Could you check a few things on this model? Use its own coordinates, in mm. A direction names the side the tool comes from. Give positions to 0.01 mm unless a question says otherwise; leave off trailing zeros. Write each loop counter-clockwise with the first axis right and the second up, starting at its lowest first coordinate (ties: lowest second). Pieces come first, ordered by that corner, then holes. Notation, with made-up numbers: (59, 73) - (111, 73) arc R31 ccw to (111, 99) - close; hole circle Ø5 at (-1.5, 28.25). An arc over 180 degrees is marked (long way). Answer as a JSON object with one key per item and string values. Group by question number.
```python
from build123d import *

# Parameters (mm, degrees)
SKETCH_1_W          = 140
SKETCH_1_H          = 55
EXTRUDE_1_DEPTH     = 12
SKETCH_2_R          = 6.5
SKETCH_2_R_2        = 4.5
CUT_EXTRUDE_1_DEPTH = 77.159372371
FILLET_1_R          = 3
SKETCH_10_R         = 7
CUT_EXTRUDE_2_DEPTH = 8
SKETCH_11_R         = 15
CUT_EXTRUDE_3_DEPTH = 8
HOLE_WIZARD_M6_1_D  = 5


with BuildPart() as part:
    # 草图1 → 凸台-拉伸1 (new body)
    with BuildSketch(Plane.XY):
        Rectangle(SKETCH_1_W, SKETCH_1_H)
    extrude(amount=EXTRUDE_1_DEPTH)

    # 草图2 → 切除-拉伸1 (cut, through all)
    with BuildSketch(Plane.XY.offset(12)):
        Circle(SKETCH_2_R)
        with Locations((-53, 0)):
            Circle(SKETCH_2_R_2)
        with Locations((53, 0)):
            Circle(SKETCH_2_R_2)
    extrude(amount=-CUT_EXTRUDE_1_DEPTH, mode=Mode.SUBTRACT)

    # 圆角1
    fillet_1_edges = [part.edges().sort_by_distance(p)[0] for p in [
        (70, -27.5, 6),
        (-70, -27.5, 6),
        (-70, 27.5, 6),
        (70, 27.5, 6),
    ]]
    fillet(fillet_1_edges, radius=FILLET_1_R)

    # 草图10 → 切除-拉伸2 (cut)
    with BuildSketch(Plane.XY.offset(12)):
        with Locations((-53, 0)):
            Circle(SKETCH_10_R)
        with Locations((53, 0)):
            Circle(SKETCH_10_R)
    extrude(amount=-CUT_EXTRUDE_2_DEPTH, mode=Mode.SUBTRACT)

    # 草图11 → 切除-拉伸3 (cut)
    with BuildSketch(Plane.XY.offset(12)):
        Circle(SKETCH_11_R)
    extrude(amount=-CUT_EXTRUDE_3_DEPTH, mode=Mode.SUBTRACT)

    # M6 螺纹孔1 (through all)
    with Locations(Plane.XY.offset(12)):
        with Locations((-60, 22.5), (-60, -22.5), (0, -22.5), (0, 22.5), (60, 22.5), (60, -22.5)):
            Hole(HOLE_WIZARD_M6_1_D / 2)


solid = part.part
```
(1) I want a section at C-C, the plane x = -53. Please give me the cut outline in (y, z).
(2) I want a section at A-A, the plane y = 22.5. Please give me the cut outline in (x, z).
(3) I want a section at D-D, the plane y = 0. Please give me the cut outline in (x, z), and give its area (3 significant figures).
(4) I want a section at B-B, the plane z = 8.5. State how many separate pieces and enclosed holes the cut face has, and give its area (3 significant figures).
(5) I need wall thicknesses on L1, parallel to Y at x = 0, z = 1.6; L2, parallel to Y at x = 0, z = 5.75; L3, parallel to Y at x = 60, z = 2.5. Which ranges of each line are inside material? Lowest first, please.
(6) Will these pins go through, and if not, where does the flat tip stop? P1, Ø8, axis at x = 50, y = 7.5, coming from the -Z side; P2, Ø4.5, axis at x = -60, y = -22.5, coming from the -Z side; P3, Ø24, axis at x = 1.5, y = 2.5, coming from the +Z side.
(7) If we mould it in two halves opening along Y, with no side actions, what happens to faces 1 (the flat face through (-1, 27.5, 6)), 2 (the cylindrical face through (58.66, -20.39, 5.92)), 3 (the cylindrical face through (69.1, -26.64, 6.08))? For each: +Y half, -Y half, draft (parallel to the pull), parting line (faces both ways), or undercut.
(8) For faces 4 (the flat face through (-53, -5, 4)), 5 (the cylindrical face through (-61.34, -20.39, 5.92)), which set-ups out of +Z, -Z, +X, -X, +Y, -Y let a thin tool reach every point of the face, with its end or its side?
Entries:
{
 "1": {"outline": "(-27.5, 0) - (-4.5, 0) - (-4.5, 4) - (-7, 4) - (-7, 12) - (-27.5, 12) - close; (4.5, 0) - (27.5, 0) - (27.5, 12) - (7, 12) - (7, 4) - (4.5, 4) - close"},
 "2": {"outline": "(-70, 0) - (-62.5, 0) - (-62.5, 12) - (-70, 12) - close; (-57.5, 0) - (-2.5, 0) - (-2.5, 12) - (-57.5, 12) - close; (2.5, 0) - (57.5, 0) - (57.5, 12) - (2.5, 12) - close; (62.5, 0) - (70, 0) - (70, 12) - (62.5, 12) - close"},
 "3": {"outline": "(-70, 0) - (-57.5, 0) - (-57.5, 4) - (-60, 4) - (-60, 12) - (-70, 12) - close; (-48.5, 0) - (-6.5, 0) - (-6.5, 4) - (-15, 4) - (-15, 12) - (-46, 12) - (-46, 4) - (-48.5, 4) - close; (6.5, 0) - (48.5, 0) - (48.5, 4) - (46, 4) - (46, 12) - (15, 12) - (15, 4) - (6.5, 4) - close; (57.5, 0) - (70, 0) - (70, 12) - (60, 12) - (60, 4) - (57.5, 4) - close", "area": "1,090 mm^2"},
 "4": {"separate pieces": "1", "enclosed holes": "9", "area": "6,560 mm^2"},
 "5": {"L1": "-27.5 to -25, -20 to -6.5, 6.5 to 20, 25 to 27.5", "L2": "-27.5 to -25, -20 to -15, 15 to 20, 25 to 27.5", "L3": "-27.5 to -25, -20 to 20, 25 to 27.5"},
 "6": {"P1": "z = 0", "P2": "through", "P3": "z = 4"},
 "7": {"face 1": "+Y half", "face 2": "undercut", "face 3": "-Y half"},
 "8": {"face 4": "+Z", "face 5": "+Z, -Z"}
}
